```python
from build123d import *

# Parameters (mm, degrees)
SKETCH1_W           = 70
SKETCH1_H           = 100
BOSS_EXTRUDE1_DEPTH = 5
SKETCH3_R           = 2.5
BOSS_EXTRUDE2_DEPTH = 20


with BuildPart() as part:
    # Sketch1 → Boss-Extrude1 (new, symmetric)
    with BuildSketch(Plane.XY):
        Rectangle(SKETCH1_W, SKETCH1_H)
    extrude(amount=BOSS_EXTRUDE1_DEPTH, both=True)

    # Sketch3 → Boss-Extrude2 (add)
    with BuildSketch(Plane.XY.offset(5)):
        with Locations(Location((0, 0, 0), (0, 0, 180))):
            Circle(SKETCH3_R)
    extrude(amount=BOSS_EXTRUDE2_DEPTH)

    # Sketch5 → Revolve1 (revolve)
    with BuildSketch(Plane(origin=(0, 0, 0), x_dir=(0, 0, -1), z_dir=(1, 0, 0))):
        Polygon((-5, 6), (-15, 6), (-15, 8), (-25, 8), (-25, 10), (-5, 10), align=None)
    revolve(axis=Axis((0, 0, 0), (0, 0, 1)))


solid = part.part
```
Here's how the part is built. I have some questions about the finished solid (model axes, mm). A direction names the side the tool comes from. Give positions to 0.01 mm unless a question says otherwise; leave off trailing zeros. Loops run counter-clockwise (first coordinate to the right, second up) from the corner with the lowest first, then second, coordinate; pieces in that order, holes last. Notation, with made-up numbers: M 14.25,5.25 L 37.25,5.25 A24 ccw 37.25,21.25 Z; hole C -30,44 d5. An arc over 180 degrees is marked long. Use one line per item in the form item = value. Start each with the question number.
Q1. If we section it at D-D (z = 20.5): Write out the boundary of the cut face in (x, y), then the cut area to 3 significant figures.
Q2. If we section it at B-B (z = 12.75): Write out the boundary of the cut face in (x, y).
Q3. Thinking about a two-plate mould opening in Y: for faces 3 (the cylindrical face through (0, -6, 10)), 4 (the flat face through (0, 1, -5)), 5 (the cylindrical face through (9.76, -2.17, 14.86)), 6 (the flat face through (3, 0, 5)), which applies, +Y half, -Y half, draft (parallel to the pull), parting line (faces both ways), or undercut?
Q4. If we section it at A-A (y = 0): Write out the boundary of the cut face in (x, z).
Q5. I need wall thicknesses on line 1 along Y through (x, z) = (0, 10); line 2 along Y through (x, z) = (0, 22.25); line 3 along Z through (x, y) = (-23, -1). Which ranges of each line are inside material? Lowest first, please.
Q6. Will these pins go through, and if not, where does the flat tip stop? pin 1 Ø5 at (x, z) = (8, 9) entering from +Y; pin 2 Ø1 at (x, y) = (-17, -7.5) entering from +Z; pin 3 Ø2 at (x, z) = (5, 14.5) entering from -Y.
Q7. Which directions (+Z, -Z, +X, -X, +Y, -Y) give clear straight access to the entire face, cutting with the end or side of a thin tool? Please do faces 1 (the flat face through (0, -50, 0)), 2 (the flat face through (-6, 2, 15)).
Q8. If we section it at C-C (x = 0): Write out the boundary of the cut face in (y, z).
Taken from the geometry:
q1.outline = C 0,0 d20; C 0,0 d5; hole C 0,0 d16
q1.area = 133 mm^2
q2.outline = C 0,0 d20; C 0,0 d5; hole C 0,0 d12
q3.face_3 = undercut
q3.face_4 = draft
q3.face_5 = parting line
q3.face_6 = undercut
q4.outline = M -35,-5 L 35,-5 L 35,5 L 10,5 L 10,25 L 8,25 L 8,15 L 6,15 L 6,5 L 2.5,5 L 2.5,25 L -2.5,25 L -2.5,5 L -6,5 L -6,15 L -8,15 L -8,25 L -10,25 L -10,5 L -35,5 Z
q5.line_1 = -10 to -6, -2.5 to 2.5, 6 to 10
q5.line_2 = -10 to -8, -2.5 to 2.5, 8 to 10
q5.line_3 = -5 to 5
q6.pin_1 = 8.35
q6.pin_2 = 5
q6.pin_3 = -9.17
q7.face_1 = +Z, -Z, +X, -X, -Y
q7.face_2 = +Z
q8.outline = M -50,-5 L 50,-5 L 50,5 L 10,5 L 10,25 L 8,25 L 8,15 L 6,15 L 6,5 L 2.5,5 L 2.5,25 L -2.5,25 L -2.5,5 L -6,5 L -6,15 L -8,15 L -8,25 L -10,25 L -10,5 L -50,5 Z
